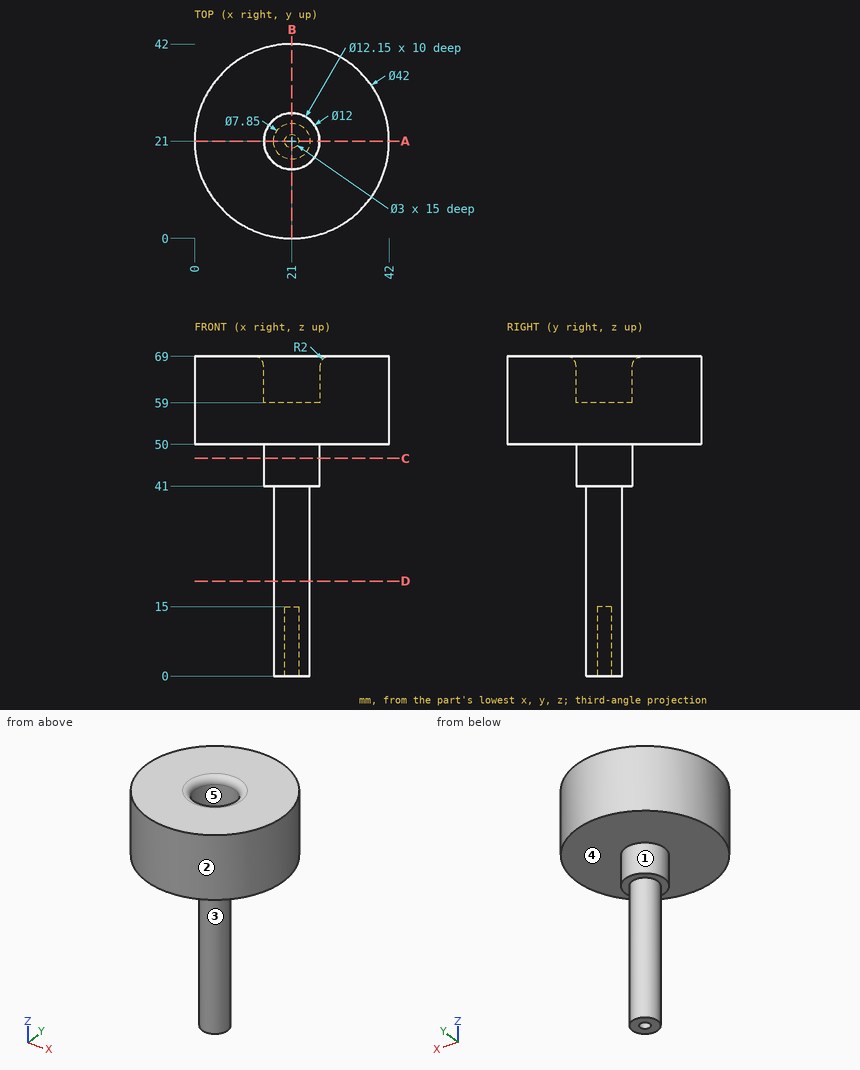
Could you check a few things on this drawing? It's one solid part, dimensions in mm from its lowest x, y, z. A direction names the side the tool comes from. Round coordinates to 2 decimals unless told otherwise and drop trailing zeros. Loops run counter-clockwise (first coordinate to the right, second up) from the corner with the lowest first, then second, coordinate; pieces in that order, holes last. Notation, with made-up numbers: M -17,7.5 L 34,7.5 A21 cw 34,20.5 Z; hole C -28.5,41.5 d1. An arc over 180 degrees is marked long. Write item = value, one per line. Start each with the question number.
(1) Suppose I cut it at C-C on z = 47. Write out the boundary of the cut face in (x, y), plus the area to 3 significant figures.
(2) I need wall thicknesses on line 1 along Y through (x, z) = (21, 5) (3 decimals); line 2 along Y through (x, z) = (21, 66) (3 decimals); line 3 along Z through (x, y) = (11.5, 3). Which ranges of each line are inside material? Lowest first, please.
(3) If we mould it in two halves opening along Y, with no side actions, what happens to the marked faces 3, 4 and 5? For each: released by +Y, released by -Y, zero draft, split by the parting line, or undercut.
(4) Suppose I cut it at A-A on y = 21. Write out the boundary of the cut face in (x, z) (3 decimals).
(5) I'm going to push flat-ended pins straight in: P1, Ø5, axis at x = 37.5, y = 13.5, coming from the -Z side; P2, Ø5, axis at y = 14.5, z = 48, coming from the +X side; P3, Ø2.5, axis at x = 21, y = 21, coming from the +Z side. Where does each tip first touch, or does it pass through?
(6) Suppose I cut it at D-D on z = 20.5. Write out the boundary of the cut face in (x, y) (3 decimals).
(7) Which directions (+Z, -Z, +X, -X, +Y, -Y) give clear straight access to the entire face, cutting with the end or side of a thin tool? Please do the marked faces 1 and 2.
Answer block:
q1.outline = C 21,21 d12
q1.area = 113 mm²
q2.line_1 = 17.075 to 19.5, 22.5 to 24.925
q2.line_2 = 0 to 14.925, 27.075 to 42
q2.line_3 = 50 to 69
q3.face_3 = split by the parting line
q3.face_4 = zero draft
q3.face_5 = undercut
q4.outline = M 0,50 L 15,50 L 15,41 L 17.075,41 L 17.075,0 L 19.5,0 L 19.5,15 L 22.5,15 L 22.5,0 L 24.925,0 L 24.925,41 L 27,41 L 27,50 L 42,50 L 42,69 L 29.075,69 A2 ccw 27.075,67 L 27.075,59 L 14.925,59 L 14.925,67 A2 ccw 12.925,69 L 0,69 Z
q5.P1 = 50
q5.P2 = 41.4
q5.P3 = 59
q6.outline = C 21,21 d7.85
q7.face_1 = -Z
q7.face_2 = +Z, -Z
